from build123d import *

# Parameters (mm, degrees)
SKETCH1_R           = 5
BOSS_EXTRUDE3_DEPTH = 6


with BuildPart() as part:
    # Sketch1 → Boss-Extrude3 (new body)
    with BuildSketch(Plane.XY):
        with BuildLine():
            ThreePointArc((0, 21.034581504), (-21.034581504, 0), (0, -21.034581504))
            ThreePointArc((0, -21.034581504), (17.584571554, -17.551352165), (32.513452001, -7.627715134))
            ThreePointArc((32.513452001, -7.627715134), (35.706726817, 0), (32.513452001, 7.627715134))
            ThreePointArc((32.513452001, 7.627715134), (17.584571554, 17.551352165), (0, 21.034581504))
        make_face()
        Circle(SKETCH1_R, mode=Mode.SUBTRACT)
    extrude(amount=BOSS_EXTRUDE3_DEPTH)


solid = part.part
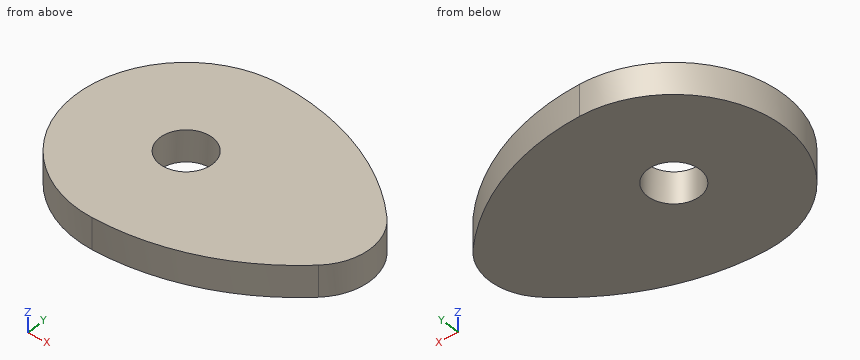
Read the model definition and answer for the solid it produces. Units are mm, in the model's axes. Coordinates: 2 decimals unless noted, no trailing zeros. Loops run counter-clockwise (first coordinate to the right, second up) from the corner with the lowest first, then second, coordinate; pieces in that order, holes last.
Q1. The part is cut by section C-C on x = -10.5. Write down the section's boundary in (y, z).
Q2. The part is cut by section A-A on y = 0. Write down the section's boundary in (x, z), and give its area (3 significant figures).
Q3. The part is cut by section B-B on z = 0.75. Write down the section's boundary in (x, y).
Q4. Each of these flat-tipped pins is pushed along its axis until it touches: pin 1 Ø2 at (x, z) = (-2, 3) entering from -Y; pin 2 Ø2 at (x, y) = (0, -10.5) entering from -Z; pin 3 Ø1.5 at (x, z) = (-12.5, 2.5) entering from +Y; pin 4 Ø2 at (y, z) = (-0.5, 1.5) entering from -X. Where does it stop, or does it pass through?
Q5. The part is cut by section D-D on y = -11. Write down the section's boundary in (x, z).
Q6. Consider probe 1 along X at (y, z) = (9, 3.1); probe 2 along X at (y, z) = (-1, 3.7); probe 3 along X at (y, z) = (-15, 0.5). Determine where each line is inside the solid, lowest interval first.
Results below:
1. outline: (-18.23, 0) - (18.23, 0) - (18.23, 6) - (-18.23, 6) - close
2. outline: (-21.03, 0) - (-5, 0) - (-5, 6) - (-21.03, 6) - close; (5, 0) - (35.71, 0) - (35.71, 6) - (5, 6) - close
2. area: 280 mm2
3. outline: (0, -21.03) arc R46.13 ccw to (32.51, -7.63) arc R10.71 ccw to (32.51, 7.63) arc R46.13 ccw to (0, 21.03) arc R21.03 ccw to start; hole circle Ø10 at (0, 0)
4. pin 1: stops at y = -21.01
4. pin 2: stops at z = 0
4. pin 3: stops at y = 17.45
4. pin 4: stops at x = -21.03
5. outline: (-17.93, 0) - (28.72, 0) - (28.72, 6) - (-17.93, 6) - close
6. probe 1: x = -19.01 to 31.07
6. probe 2: x = -21.01 to -4.9, 4.9 to 35.66
6. probe 3: x = -14.75 to 22.81
